Work out the finished part from the listing and answer in its coordinate system (mm). A direction names the side the tool comes from. Round coordinates to 2 decimals unless told otherwise and drop trailing zeros. Order: outer loops, then holes, each group sorted by start corner. A loop starts at its lowest first (then second) coordinate and runs counter-clockwise, first axis right, second up. Notation, with made-up numbers: (8.5, 1) - (15.5, 1) arc R19 ccw to (15.5, 34) - close; hole circle Ø4 at (65, 69.5). An arc over 180 degrees is marked (long way). Use one line per item in the form item = value. Start each with the question number.
Q1. The part is cut by section A-A on z = 0. Determine the outline of the cut face in (x, y), plus the area to 3 significant figures.
Q2. The part is cut by section C-C on y = 2.5. Determine the outline of the cut face in (x, z).
Q3. The part is cut by section D-D on x = 6.25. Determine the outline of the cut face in (y, z), plus the area to 3 significant figures.
Q4. Given P1, Ø1.9, axis at y = 17, z = -0.5, coming from the +X side, flat-ended and moving along its own axis, determine where the tip first touches the part or whether it passes through.
Q5. The part is cut by section B-B on x = 0. Determine the outline of the cut face in (y, z).
Q6. For a pull along X with two mould halves and no side action, classify faces 4 (the cylindrical face through (7.634, 12.675, 0.683)), 5 (the flat face through (-2, 3, 1.5)), 6 (the flat face through (5.2, 16, 0)), 7 (the flat face through (-3, 3, -1.5)) as +X half, -X half, draft (parallel to the pull), parting line (faces both ways), or undercut.
Q7. Which of the six approach directions +Z, -Z, +X, -X, +Y, -Y give full straight-line access (tool end or side, diameter ignored) to faces 1 (the flat face through (8, 22.5, 0)), 2 (the flat face through (5, 14, 0)), 3 (the cylindrical face through (-8.5, 2.5, 0))?
Q8. Find the intervals of material crossed by line 1 (X direction, y = 4, z = 0); line 2 (Y direction, x = 7, z = 0); line 3 (X direction, y = 6.5, z = -3.5), in increasing order. Write a range as [from, to].
from build123d import *

# Parameters (mm, degrees)
CROQUIS1_W              = 20
CROQUIS1_H              = 15
SALIENTE_EXTRUIR1_DEPTH = 5
CROQUIS2_W              = 5
CROQUIS2_H              = 15
SALIENTE_EXTRUIR2_DEPTH = 21.5
CROQUIS3_R              = 3.15
CORTAR_EXTRUIR1_DEPTH   = 20
CORTAR_EXTRUIR2_DEPTH   = 20
CROQUIS7_R              = 4
SALIENTE_EXTRUIR3_DEPTH = 0.2
CROQUIS8_W              = 15
CROQUIS8_H              = 4
CORTAR_EXTRUIR3_DEPTH   = 10


with BuildPart() as part:
    # Croquis1 → Saliente-Extruir1 (new body)
    with BuildSketch(Plane(origin=(0, 0, 0), x_dir=(1, 0, 0), z_dir=(0, 1, 0))):
        Rectangle(CROQUIS1_W, CROQUIS1_H)
    extrude(amount=SALIENTE_EXTRUIR1_DEPTH)

    # Croquis2 → Saliente-Extruir2 (add)
    with BuildSketch(Plane(origin=(0, 5, 0), x_dir=(1, 0, 0), z_dir=(0, 1, 0))):
        with Locations((7.5, 0)):
            Rectangle(CROQUIS2_W, CROQUIS2_H)
    extrude(amount=SALIENTE_EXTRUIR2_DEPTH)

    # Croquis3 → Cortar-Extruir1 (cut)
    with BuildSketch(Plane(origin=(10, 0, 0), x_dir=(0, 0, -1), z_dir=(1, 0, 0))):
        with Locations((0, 15.75)):
            Circle(CROQUIS3_R)
    extrude(amount=-CORTAR_EXTRUIR1_DEPTH, mode=Mode.SUBTRACT)

    # Croquis4 → Cortar-Extruir2 (cut)
    with BuildSketch(Plane(origin=(0, 5, 0), x_dir=(1, 0, 0), z_dir=(0, 1, 0))):
        with BuildLine():
            Line((-7, 1.5), (2, 1.5))
            ThreePointArc((2, 1.5), (3.5, 0), (2, -1.5))
            Line((2, -1.5), (-7, -1.5))
            ThreePointArc((-7, -1.5), (-8.5, 0), (-7, 1.5))
        make_face()
    extrude(amount=-CORTAR_EXTRUIR2_DEPTH, mode=Mode.SUBTRACT)

    # Croquis7 → Saliente-Extruir3 (add)
    with BuildSketch(Plane.ZY.offset(-5)):
        with Locations((0, 15.75)):
            Circle(CROQUIS7_R)
    extrude(amount=-SALIENTE_EXTRUIR3_DEPTH)

    # Croquis8 → Cortar-Extruir3 (cut)
    with BuildSketch(Plane(origin=(10, 0, 0), x_dir=(0, 0, -1), z_dir=(1, 0, 0))):
        with Locations((0, 24.5)):
            Rectangle(CROQUIS8_W, CROQUIS8_H)
    extrude(amount=-CORTAR_EXTRUIR3_DEPTH, mode=Mode.SUBTRACT)


solid = part.part
Found:
q1.outline = (-10, 0) - (-8.5, 0) - (-8.5, 5) - (-10, 5) - close; (3.5, 0) - (10, 0) - (10, 12.6) - (5.2, 12.6) - (5.2, 18.9) - (10, 18.9) - (10, 22.5) - (5, 22.5) - (5, 5) - (3.5, 5) - close
q1.area = 97.3 mm²
q2.outline = (-10, -7.5) - (10, -7.5) - (10, 7.5) - (-10, 7.5) - close; hole (-7, -1.5) - (2, -1.5) arc R1.5 ccw to (2, 1.5) - (-7, 1.5) arc R1.5 ccw to start
q3.outline = (0, -7.5) - (22.5, -7.5) - (22.5, 7.5) - (0, 7.5) - close; hole circle Ø6.3 at (15.75, 0)
q3.area = 306 mm²
q4.P1 = 5.2
q5.outline = (0, -7.5) - (5, -7.5) - (5, -1.5) - (0, -1.5) - close; (0, 1.5) - (5, 1.5) - (5, 7.5) - (0, 7.5) - close
q6.face_4 = draft
q6.face_5 = undercut
q6.face_6 = +X half
q6.face_7 = undercut
q7.face_1 = +Z, -Z, +X, -X, +Y
q7.face_2 = +Z, -Z, -X, +Y
q7.face_3 = +Y, -Y
q8.line_1 = [-10, -8.5], [3.5, 10]
q8.line_2 = [0, 12.6], [18.9, 22.5]
q8.line_3 = [5, 10]
